Geometry: see drawing. Coordinates: mm, zero at the bounding-box minimum. Round coordinates to 2 decimals unless told otherwise and drop trailing zeros. Loops run counter-clockwise (first coordinate to the right, second up) from the corner with the lowest first, then second, coordinate; pieces in that order, holes last.
(1) Cut plane A-A, the plane x = 26. Output: boundary loops of the cut face in (y, z), and give its area (3 significant figures).
(2) Cut plane D-D, the plane y = 5. Output: boundary loops of the cut face in (x, z), and give its area (3 significant figures).
(3) Cut plane C-C, the plane y = 1.75. Output: boundary loops of the cut face in (x, z).
(4) Draft query along Y for the marked faces 1, 2 and 3. Return one class per face: released by +Y, released by -Y, zero draft, split by the parting line, or undercut.
(5) Cut plane B-B, the plane z = 1.15. Output: boundary loops of the cut face in (x, y).
(6) Line query: line 1 (Y direction, x = 10, z = 1.05); line 2 (X direction, y = 1.25, z = 0.3); line 3 (X direction, y = 16.75, z = 0.85). Output: solid intervals per line, ascending.
(7) First-contact query: pin 1 Ø2.5 at (x, y) = (26, 17.5) entering from +Z; pin 2 Ø0.9 at (y, z) = (15, 1.5) entering from -X; pin 3 Ø0.8 at (x, z) = (1.5, 1) entering from +Y. Flat tips, straight axial feed; report the tip coordinate or a pass-through.
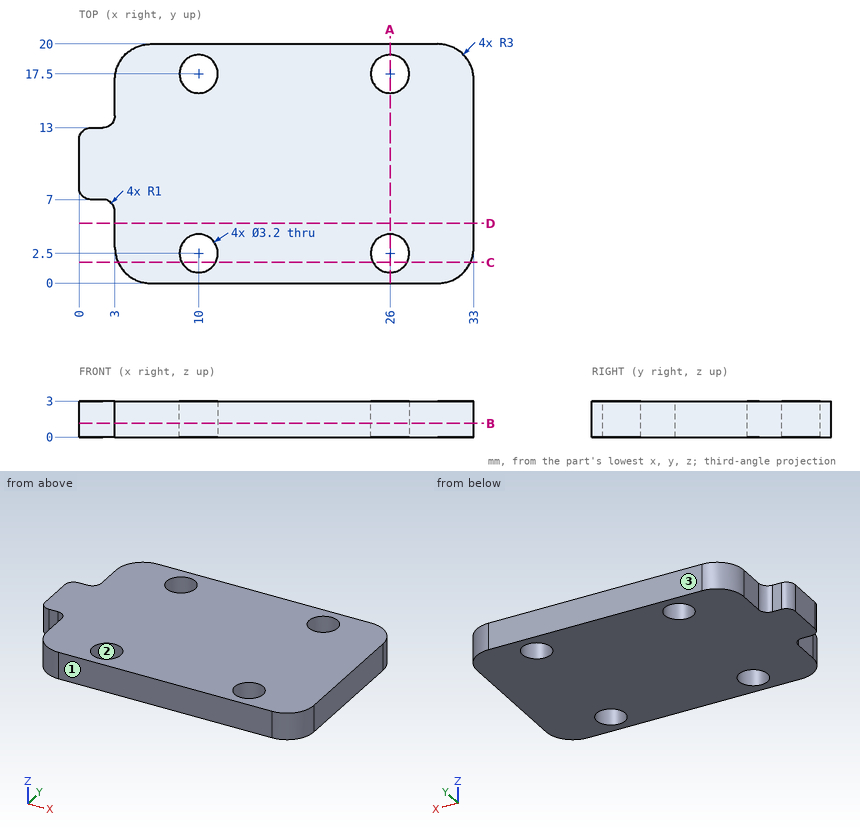
Reported:
1. outline: (0, 0) - (0.9, 0) - (0.9, 3) - (0, 3) - close; (4.1, 0) - (15.9, 0) - (15.9, 3) - (4.1, 3) - close; (19.1, 0) - (20, 0) - (20, 3) - (19.1, 3) - close
1. area: 40.8 mm2
2. outline: (3, 0) - (33, 0) - (33, 3) - (3, 3) - close
2. area: 90.0 mm2
3. outline: (3.27, 0) - (8.59, 0) - (8.59, 3) - (3.27, 3) - close; (11.41, 0) - (24.59, 0) - (24.59, 3) - (11.41, 3) - close; (27.41, 0) - (32.73, 0) - (32.73, 3) - (27.41, 3) - close
4. face 1: released by -Y
4. face 2: undercut
4. face 3: released by +Y
5. outline: (0, 8) arc R1 ccw to (1, 7) - (2, 7) arc R1 cw to (3, 6) - (3, 3) arc R3 ccw to (6, 0) - (30, 0) arc R3 ccw to (33, 3) - (33, 17) arc R3 ccw to (30, 20) - (6, 20) arc R3 ccw to (3, 17) - (3, 14) arc R1 cw to (2, 13) - (1, 13) arc R1 ccw to (0, 12) - close; hole circle Ø3.2 at (10, 2.5); hole circle Ø3.2 at (10, 17.5); hole circle Ø3.2 at (26, 2.5); hole circle Ø3.2 at (26, 17.5)
6. line 1: y = 0 to 0.9, 4.1 to 15.9, 19.1 to 20
6. line 2: x = 3.56 to 9, 11 to 25, 27 to 32.44
6. line 3: x = 3 to 8.59, 11.41 to 24.59, 27.41 to 33
7. pin 1: passes through
7. pin 2: stops at x = 3
7. pin 3: stops at y = 13
